Autodesk Inventor part; units mm, degrees
ref_plane "YZ Plane" through (0, 0, 0) normal (1, 0, 0) x (0, 1, 0)
ref_plane "XZ Plane" through (0, 0, 0) normal (0, 1, 0) x (-1, 0, 0)
ref_plane "XY Plane" through (0, 0, 0) normal (0, 0, 1) x (1, 0, 0)
sketch "スケッチ1" plane through (0, 0, 0) normal (0, 1, 0) x (-1, 0, 0)
  line L0 (-2, 11) -> (2, 11)
  line L1 (2, 11) -> (2, -11)
  line L2 (2, -11) -> (-2, -11)
  line L3 (-2, -11) -> (-2, 11)
  line L4 (-2, 11) -> (2, -11) construction
  line L5 (2, 11) -> (-2, -11) construction
  circle A0 centre (0, 8.5) radius 0.8
  line L6 (0, -15.4) -> (0, 15.4) construction
  circle A1 centre (0, -8.5) radius 0.8
  line L7 (2.8, 0) -> (-2.8, 0)
  point P0 (0, 0)
  dimension "d0" = 4
  dimension "d1" = 2.5
  dimension "d2" = 1.6
  dimension "d3" = 22
extrude "押し出し1" add sketch "スケッチ1" along normal blind 4
sketch "スケッチ2" plane through (0, 4, 0) normal (0, 1, 0) x (1, 0, 0)
  line L0 (5, -15) -> (-5, -15)
  line L1 (-5, -15) -> (-5, 15)
  line L2 (-5, 15) -> (5, 15)
  line L3 (5, 15) -> (5, -15)
  line L4 (5, -15) -> (-5, 15) construction
  line L5 (-5, -15) -> (5, 15) construction
  line L6 (2, -11) -> (2, 11)
  line L7 (2, 11) -> (-2, 11)
  line L8 (-2, 11) -> (-2, -11)
  line L9 (-2, -11) -> (2, -11)
  circle A0 centre (0, 8.5) radius 0.8
  circle A1 centre (0, -8.5) radius 0.8
  point P0 (0, 0)
  dimension "d6" = 30
  dimension "d7" = 10
extrude "押し出し2" add sketch "スケッチ2" along normal blind 3 contours L0 L1 L2 L3 | L9 L8 L7 L6
properties part number "Zigu"
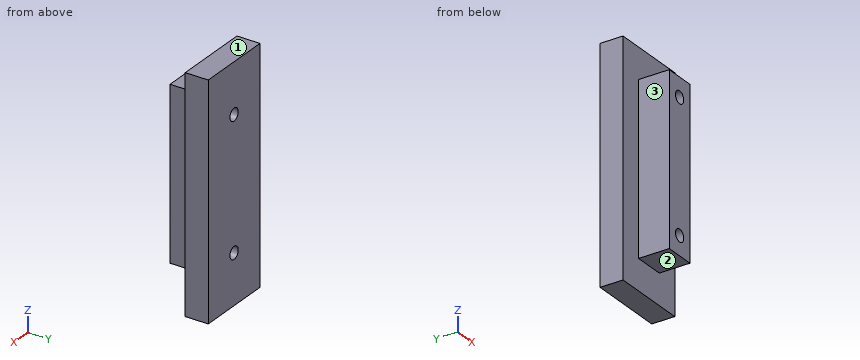
The model under review builds one solid part; all positions refer to its coordinate system, in mm. Face numbers are marked on the shaded views. A direction names the side the tool comes from. Round coordinates to 2 decimals unless told otherwise and drop trailing zeros. Write each loop counter-clockwise with the first axis right and the second up, starting at its lowest first coordinate (ties: lowest second). Pieces come first, ordered by that corner, then holes. Notation, with made-up numbers: (66.5, -28) -> (98.5, -28) arc R16 ccw to (98.5, -9) -> close; hole circle Ø10 at (65.25, 83). An arc over 180 degrees is marked (long way). Use CSV: the item, a comma, the result in double quotes.
Q1. For pin 1 Ø1 at (x, y) = (-2, 2) entering from +Z; pin 2 Ø1.2 at (y, z) = (2, 1) entering from -X; pin 3 Ø3 at (x, y) = (0, 1) entering from -Z, all flat-tipped, find the tip position at first contact; note any pin that passes through.
Checks:
pin 1,"z = 11"
pin 2,"x = -2"
pin 3,"z = -11"
Q2. Consider section C-C (z = 10). Give the boundary of the cut face in (x, y), then the cut area to 3 significant figures.
Checks:
outline,"(-5, 4) -> (-2, 4) -> (-2, 0) -> (2, 0) -> (2, 4) -> (5, 4) -> (5, 7) -> (-5, 7) -> close"
area,"46.0 mm²"
Q3. For the marked faces 1, 2 and 3, list the 3-axis set-ups (+Z, -Z, +X, -X, +Y, -Y) from which the entire face can be reached by the end or side of a thin tool; tool diameter is ignored.
Checks:
face 1,"+Z, +X, -X, +Y, -Y"
face 2,"-Z, +X, -X, -Y"
face 3,"+Z, -Z, -X, -Y"
Q4. To check wall thickness, follow probe 1 along Z at (x, y) = (0, 4.25); probe 2 along Z at (x, y) = (0.25, 0.5); probe 3 along X at (y, z) = (3.5, -8.5). State the ranges of each line that lie inside material, in increasing order. Write a range as [from, to].
Checks:
probe 1,"[-15, -9.3], [-7.7, 7.7], [9.3, 15]"
probe 2,"[-11, -9.26], [-7.74, 7.74], [9.26, 11]"
probe 3,"[-2, -0.8], [0.8, 2]"
Q5. Consider section D-D (x = 3). Give the boundary of the cut face in (y, z).
Checks:
outline,"(4, -15) -> (7, -15) -> (7, 15) -> (4, 15) -> close"
Q6. Consider section A-A (y = 0.75). Give the boundary of the cut face in (x, z).
Checks:
outline,"(-2, -11) -> (2, -11) -> (2, 11) -> (-2, 11) -> close; hole circle Ø1.6 at (0, -8.5); hole circle Ø1.6 at (0, 8.5)"
